Source: three-view drawing plus pictorial views. Frame: mm from the lowest corner of the part. Round coordinates to 2 decimals unless told otherwise and drop trailing zeros. Loops run counter-clockwise (first coordinate to the right, second up) from the corner with the lowest first, then second, coordinate; pieces in that order, holes last. Notation, with made-up numbers: M -6.5,-6.5 L 12.5,-6.5 A10 cw 12.5,-1.5 Z; hole C 20.25,56 d8. An arc over 180 degrees is marked long. Return JSON: item names as keys, results as strings. Group by question number.
1) Section D-D (x = 5.3). Output: boundary loops of the cut face in (y, z), plus the area to 3 significant figures.
2) Contact query for flat-ended pins moving along their axis: P1, Ø0.8, axis at x = 3.5, y = 2.5, coming from the -Z side; P2, Ø1.5, axis at y = 1, z = 46.5, coming from the -X side. Output: stop coordinate, or through.
3) Section C-C (z = 16). Output: boundary loops of the cut face in (x, y), plus the area to 3 significant figures.
4) Material intervals for line 1 (Y direction, x = 3, z = 2.6); line 2 (Z direction, x = 2.5, y = 3.7); line 3 (Y direction, x = 1.2, z = 29.5), sorted ascending. Write a range as from..to.
5) Section A-A (y = 3). Output: boundary loops of the cut face in (x, z).
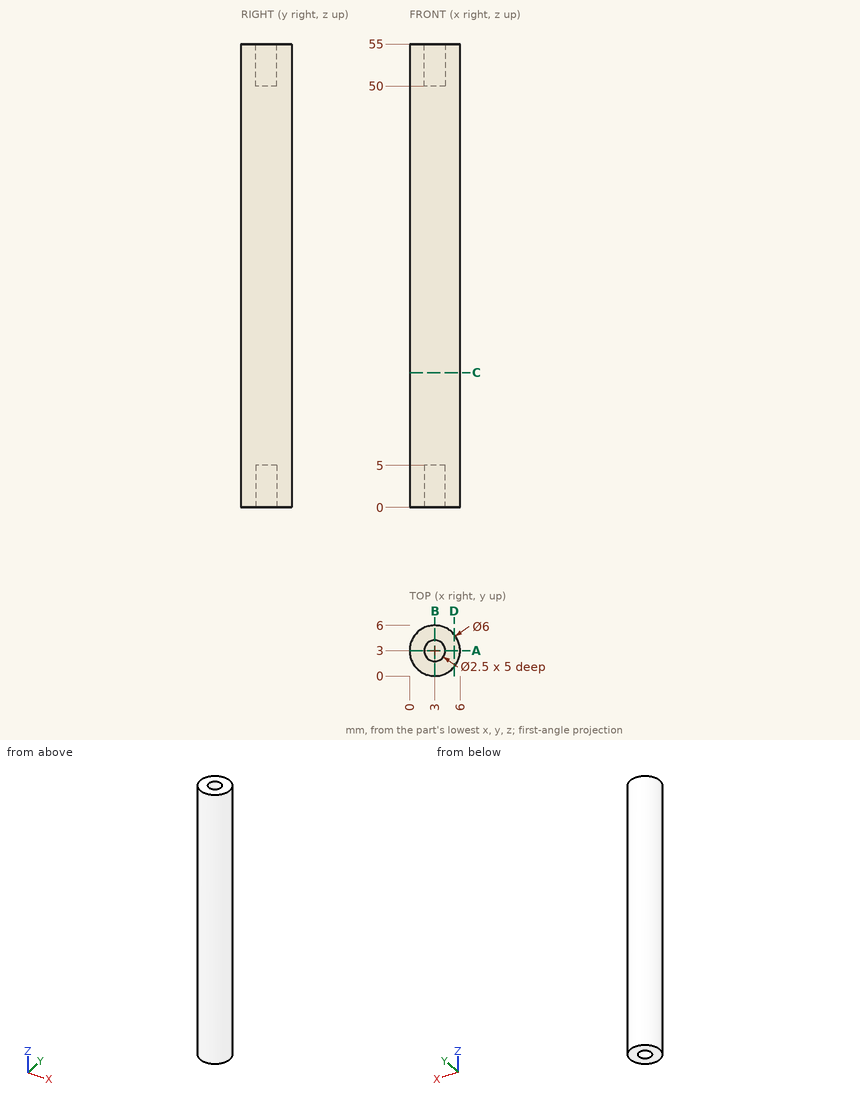
Returned:
{
 "1": {"outline": "M 1.07,0 L 4.93,0 L 4.93,55 L 1.07,55 Z", "area": "212 mm^2"},
 "2": {"P1": "stops at z = 5", "P2": "stops at x = 0.27"},
 "3": {"outline": "C 3,3 d6", "area": "28.3 mm^2"},
 "4": {"line 1": "y = 0..1.75, 4.25..6", "line 2": "z = 5..50", "line 3": "y = 0.6..5.4"},
 "5": {"outline": "M 0,0 L 1.75,0 L 1.75,5 L 4.25,5 L 4.25,0 L 6,0 L 6,55 L 4.25,55 L 4.25,50 L 1.75,50 L 1.75,55 L 0,55 Z"}
}
